Read the model definition and answer for the solid it produces. Units are mm, in the model's axes. A direction names the side the tool comes from. Coordinates: 2 decimals unless noted, no trailing zeros. Loops run counter-clockwise (first coordinate to the right, second up) from the corner with the lowest first, then second, coordinate; pieces in that order, holes last. Notation, with made-up numbers: (-11, -18) - (34, -18) arc R16 ccw to (34, 5) - close; hole circle Ø9 at (-33, 78.25). An arc over 180 degrees is marked (long way). One line per question, with ' | ' between items. Start each with the question number.
```python
from build123d import *

# Parameters (mm, degrees)
SKETCH1_R           = 1.7
BOSS_EXTRUDE1_DEPTH = 2


with BuildPart() as part:
    # Sketch1 → Boss-Extrude1 (new body)
    with BuildSketch(Plane(origin=(0, 2, 0), x_dir=(1, 0, 0), z_dir=(0, 1, 0))):
        with BuildLine():
            Line((26.292893219, -7.207106781), (27.707106781, -5.792893219))
            ThreePointArc((27.707106781, -5.792893219), (27.923879533, -5.46846987), (28, -5.085786438))
            Line((28, -5.085786438), (28, 5.085786438))
            ThreePointArc((28, 5.085786438), (27.923879533, 5.46846987), (27.707106781, 5.792893219))
            Line((27.707106781, 5.792893219), (26.292893219, 7.207106781))
            ThreePointArc((26.292893219, 7.207106781), (25.96846987, 7.423879533), (25.585786438, 7.5))
            Line((25.585786438, 7.5), (-2.3, 7.5))
            ThreePointArc((-2.3, 7.5), (-3.007106781, 7.207106781), (-3.3, 6.5))
            Line((-3.3, 6.5), (-3.3, 5))
            ThreePointArc((-3.3, 5), (-3.797918472, 3.797918472), (-5, 3.3))
            Line((-5, 3.3), (-6.5, 3.3))
            ThreePointArc((-6.5, 3.3), (-7.207106781, 3.007106781), (-7.5, 2.3))
            Line((-7.5, 2.3), (-7.5, -25.585786438))
            ThreePointArc((-7.5, -25.585786438), (-7.423879533, -25.96846987), (-7.207106781, -26.292893219))
            Line((-7.207106781, -26.292893219), (-5.792893219, -27.707106781))
            ThreePointArc((-5.792893219, -27.707106781), (-5.46846987, -27.923879533), (-5.085786438, -28))
            Line((-5.085786438, -28), (5.085786438, -28))
            ThreePointArc((5.085786438, -28), (5.46846987, -27.923879533), (5.792893219, -27.707106781))
            Line((5.792893219, -27.707106781), (7.207106781, -26.292893219))
            ThreePointArc((7.207106781, -26.292893219), (7.423879533, -25.96846987), (7.5, -25.585786438))
            Line((7.5, -25.585786438), (7.5, -17.914213562))
            ThreePointArc((7.5, -17.914213562), (7.576120467, -17.53153013), (7.792893219, -17.207106781))
            Line((7.792893219, -17.207106781), (17.207106781, -7.792893219))
            ThreePointArc((17.207106781, -7.792893219), (17.53153013, -7.576120467), (17.914213562, -7.5))
            Line((17.914213562, -7.5), (25.585786438, -7.5))
            ThreePointArc((25.585786438, -7.5), (25.96846987, -7.423879533), (26.292893219, -7.207106781))
        make_face()
        with Locations(Location((0, -16, 0), (0, 0, 90))):
            Circle(SKETCH1_R, mode=Mode.SUBTRACT)
        with Locations(Location((0, -24, 0), (0, 0, 90))):
            Circle(SKETCH1_R, mode=Mode.SUBTRACT)
        with Locations(Location((24, 0, 0), (0, 0, 90))):
            Circle(SKETCH1_R, mode=Mode.SUBTRACT)
        with Locations(Location((16, 0, 0), (0, 0, 90))):
            Circle(SKETCH1_R, mode=Mode.SUBTRACT)
        with Locations(Location((0, 0, 0), (0, 0, 90))):
            Circle(SKETCH1_R, mode=Mode.SUBTRACT)
        with Locations(Location((8, 0, 0), (0, 0, 90))):
            Circle(SKETCH1_R, mode=Mode.SUBTRACT)
        with Locations(Location((0, -8, 0), (0, 0, 90))):
            Circle(SKETCH1_R, mode=Mode.SUBTRACT)
        with BuildLine():
            Line((4.454772721, -6.858935778), (3.797918472, -6.202081528))
            ThreePointArc((3.797918472, -6.202081528), (3.797918472, -3.797918472), (6.202081528, -3.797918472))
            Line((6.202081528, -3.797918472), (6.858935778, -4.454772721))
            ThreePointArc((6.858935778, -4.454772721), (6.858935778, -6.858935778), (4.454772721, -6.858935778))
        make_face(mode=Mode.SUBTRACT)
    extrude(amount=-BOSS_EXTRUDE1_DEPTH)


solid = part.part
```
1) The part is cut by section A-A on z = 16. Write down the section's boundary in (x, y), and give its area (3 significant figures).
2) The part is cut by section C-C on y = 0.75. Count the separate pieces of the cut face and the enclosed holes in it, and give its area (3 significant figures).
3) The part is cut by section D-D on x = -1. Write down the section's boundary in (y, z).
4) Which of the six approach directions +Z, -Z, +X, -X, +Y, -Y give full straight-line access (tool end or side, diameter ignored) to faces 5 (the flat face through (22, 1, 7.5)), 6 (the flat face through (-6, 1, -3.3)), 7 (the flat face through (27, 1, -6.5))?
5) Find the intervals of material crossed by line 1 along X through (y, z) = (0.65, 0); line 2 along Z through (x, y) = (24, 1.2); line 3 along X through (y, z) = (0.85, -1), in increasing order. Write a range as from..to.
6) The part is cut by section B-B on x = 16. Write down the section's boundary in (y, z), and give its area (3 significant figures).
7) The mould has two halves that part along X. Classify faces 1 (the flat face through (-3.3, 1, -6)), 2 (the flat face through (7.5, 1, 22)), 3 (the flat face through (0, 1, 28)), 4 (the cylindrical face through (-0.51, 1.01, 14.38)): released by +X, released by -X, zero draft, split by the parting line, or undercut.
8) Given pin 1 Ø0.8 at (y, z) = (1, -5.5) entering from -X; pin 2 Ø3 at (x, z) = (0, 8) entering from -Y; pin 3 Ø1 at (y, z) = (1.5, 16.5) entering from +X, each flat-ended and moving along its own axis, determine where each tip first touches the part or whether it passes through.
Answer below:
1) outline: (-7.5, 0) - (-1.7, 0) - (-1.7, 2) - (-7.5, 2) - close; (1.7, 0) - (9, 0) - (9, 2) - (1.7, 2) - close | area: 26.2 mm2
2) separate pieces: 1 | enclosed holes: 8 | area: 789 mm2
3) outline: (0, -7.5) - (2, -7.5) - (2, -1.37) - (0, -1.37) - close; (0, 1.37) - (2, 1.37) - (2, 6.63) - (0, 6.63) - close; (0, 9.37) - (2, 9.37) - (2, 14.63) - (0, 14.63) - close; (0, 17.37) - (2, 17.37) - (2, 22.63) - (0, 22.63) - close; (0, 25.37) - (2, 25.37) - (2, 28) - (0, 28) - close
4) face 5: +Z, +X, +Y, -Y | face 6: -Z, -X, +Y, -Y | face 7: -Z, +X, +Y, -Y
5) line 1: -7.5..-1.7, 1.7..6.3, 9.7..14.3, 17.7..22.3, 25.7..28 | line 2: -7.5..-1.7, 1.7..7.5 | line 3: -7.5..-1.37, 1.37..6.63, 9.37..14.63, 17.37..22.63, 25.37..28
6) outline: (0, -7.5) - (2, -7.5) - (2, -1.7) - (0, -1.7) - close; (0, 1.7) - (2, 1.7) - (2, 9) - (0, 9) - close | area: 26.2 mm2
7) face 1: released by -X | face 2: released by +X | face 3: zero draft | face 4: undercut
8) pin 1: x = -3.3 | pin 2: through | pin 3: x = 9
